Here's how the part is built. I have some questions about the finished solid (model axes, mm). A direction names the side the tool comes from. Round coordinates to 2 decimals unless told otherwise and drop trailing zeros. Order: outer loops, then holes, each group sorted by start corner. A loop starts at its lowest first (then second) coordinate and runs counter-clockwise, first axis right, second up. Notation, with made-up numbers: (25.5, 48.5) - (76.5, 48.5) arc R15 cw to (76.5, 74.5) - close; hole circle Ø2 at (43, 29.5). An arc over 180 degrees is marked (long way). Answer as a JSON object with one key per item and string values.
```python
from build123d import *

# Parameters (mm, degrees)
CIRPATTERN1_COUNT   = 12
CUT_EXTRUDE1_DEPTH  = 4.572
SKETCH7_W           = 1.524
SKETCH7_H           = 1.524
CUT_EXTRUDE2_DEPTH  = 9.525
BOSS_EXTRUDE1_REACH = 65.5
SKETCH8_R           = 12.7


with BuildPart() as part:
    # Sketch1 → Revolve2 (revolve)
    with BuildSketch(Plane.XY):
        with BuildLine():
            add(Edge.make_bspline(
                [(0, 48.26), (-26.035, 48.26), (-26.035, 0)],
                knots=[3.141592654, 3.141592654, 3.141592654, 4.71238898, 4.71238898, 4.71238898], degree=2, weights=[1, 0.707106781, 1]))
            Line((-26.035, 0), (-15.875, 0))
            add(Edge.make_bspline(
                [(0, 38.1), (-15.875, 38.1), (-15.875, 0)],
                knots=[3.141592654, 3.141592654, 3.141592654, 4.71238898, 4.71238898, 4.71238898], degree=2, weights=[1, 0.707106781, 1]))
            Line((0, 38.1), (0, 48.26))
        make_face()
    revolve(axis=Axis((-26.035, 0, 0), (1, 0, 0)))

    # Sketch2 → Cut-Loft1 section 0
    with BuildSketch(Plane(origin=(0, -34.29, 0), x_dir=(1, 0, 0), z_dir=(0, 1, 0)), mode=Mode.PRIVATE) as cut_loft1_s0:
        Polygon((0, 7.69896584), (-6.6675, -3.84948292), (6.6675, -3.84948292), align=None)
    cut_loft1 = loft([cut_loft1_s0.sketch, Vertex(0, -45.212, 0)], mode=Mode.SUBTRACT)

    # CirPattern1: Cut-Loft1 ×12 about axis
    cirpattern1_axis = Axis((0, 0, 0), (1, 0, 0))
    for i in range(1, CIRPATTERN1_COUNT):
        add(cut_loft1.rotate(cirpattern1_axis, i * 360 / CIRPATTERN1_COUNT), mode=Mode.SUBTRACT)


with BuildPart() as body_2:
    # Mirror5: mirrored copy
    add(part.part.mirror(Plane(origin=(0, 0, 0), x_dir=(0, 0, 1), z_dir=(1, 0, 0))))

    # Sketch6 → Cut-Extrude1 (cut)
    with BuildSketch(Plane(origin=(0, 0, 0), x_dir=(0, 0, -1), z_dir=(1, 0, 0))):
        Polygon((4.851243253, 42.407942289), (14.134652823, 40.27629228), (14.475716824, 41.761637811), (5.192307254, 43.89328782), align=None)
    cut_extrude1 = extrude(amount=CUT_EXTRUDE1_DEPTH, mode=Mode.SUBTRACT)

    # Sketch7 → Cut-Extrude2 (cut)
    with BuildSketch(Plane(origin=(0, -1.065825004, -4.641704785), x_dir=(1, 0, 0), z_dir=(0, 0.223795276, 0.974636175))):
        with Locations((3.81, 41.656)):
            Rectangle(SKETCH7_W, SKETCH7_H)
    cut_extrude2 = extrude(amount=CUT_EXTRUDE2_DEPTH, mode=Mode.SUBTRACT)

    # Mirror6: Cut-Extrude1, Cut-Extrude2 across plane
    add(cut_extrude1.mirror(Plane(origin=(0, 0, 0), x_dir=(0, 0.223795276, 0.974636175), z_dir=(0, -0.974636175, 0.223795276))), mode=Mode.SUBTRACT)
    add(cut_extrude2.mirror(Plane(origin=(0, 0, 0), x_dir=(0, 0.223795276, 0.974636175), z_dir=(0, -0.974636175, 0.223795276))), mode=Mode.SUBTRACT)

    # Sketch8 → Boss-Extrude1 (add, up to next)
    with BuildSketch(Plane(origin=(63.5, 0, 0), x_dir=(0, 0, -1), z_dir=(1, 0, 0)), mode=Mode.PRIVATE) as boss_extrude1_sk1:
        Circle(SKETCH8_R)
    boss_extrude1_tool1 = extrude(boss_extrude1_sk1.sketch, amount=-BOSS_EXTRUDE1_REACH, mode=Mode.PRIVATE) - body_2.part
    add(boss_extrude1_tool1.solids().sort_by_distance((63.5, 0, 0))[0])


solid = body_2.part
```
1. If I drill on L1, parallel to Z at x = 7, y = -7; L2, parallel to Z at x = 4, y = 14; L3, parallel to Y at x = 7, z = -16, over which ranges is the centre line in solid material (lowest first)? Write a range as [from, to].
Responses:
{"L1": "[-45.95, -33.47], [33.47, 45.95]", "L2": "[-45.59, -34.11], [34.11, 45.59]", "L3": "[-43.64, -30.22], [30.22, 43.64]"}
2. Imagine slicing it at A-A (x = 59.5). List the corners of the cut face in (y, z) for me, plus the area to 3 significant figures.
Responses:
{"outline": "circle Ø25.4 at (0, 0)", "area": "507 mm2"}
3. For faces 1 (the face through (1.503, -41.327, 9.558)), 2 (the face through (4.572, 41, -9)), which set-ups out of +Z, -Z, +X, -X, +Y, -Y let a thin tool reach every point of the face, with its end or its side?
Responses:
{"face 1": "-X", "face 2": "none"}
4. For P1, Ø3, axis at y = 13, z = -1.5, coming from the -X side; P2, Ø4, axis at x = 16, y = 30, coming from the +Z side; P3, Ø1.8, axis at y = -41.5, z = 11.5, coming from the +X side, each with a flat end and sliding along its axis, tell me the tip position at first contact or that it passes through.
Responses:
{"P1": "x = 14.67", "P2": "z = 28.08", "P3": "x = 12.67"}
5. Thinking about a two-plate mould opening in Y: for faces 3 (the face through (44.58, -12.4, 2.75)), 4 (the face through (2.011, 34.482, -19.286)), which applies, pulls with the +Y half, pulls with the -Y half, needs draft (parallel to the pull), parting line crosses it, or undercut?
Responses:
{"face 3": "parting line crosses it", "face 4": "undercut"}
